```python
from build123d import *

# Parameters (mm, degrees)
F0_R     = 17.5
F0_R_2   = 15.5
F1_DEPTH = 6
F2_R     = 20
F3_DEPTH = 2
F4_SIZE  = 2.49999


# Not quite as in the source:
# - a fillet or chamfer is up to 0.001 mm smaller than in the source, because OpenCascade refuses the exact size


with BuildPart() as f1:
    # F0 (on Top) → F1 (new body)
    with BuildSketch(Plane.XY):
        Circle(F0_R)
        Circle(F0_R_2, mode=Mode.SUBTRACT)
    extrude(amount=F1_DEPTH)

    # F2 (on Top) → F3 (join)
    with BuildSketch(Plane.XY):
        Circle(F2_R)
    extrude(amount=F3_DEPTH)

    # F4 (size 2.5 in the source; OpenCascade refuses exactly that, so slightly less here)
    f4_edges = [f1.edges().sort_by_distance(p)[0] for p in [
        (-17.5, 0, 2),
    ]]
    chamfer(f4_edges, length=F4_SIZE)


solid = f1.part
```
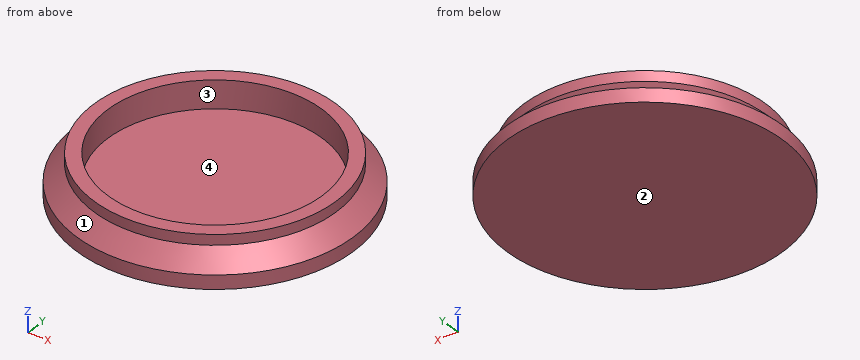
The listing builds one solid part. Answer for the finished solid, in the listing's coordinates (mm). Face numbers are marked on the shaded views. Give positions to 0.01 mm unless a question says otherwise; leave off trailing zeros. Order: outer loops, then holes, each group sorted by start corner. A loop starts at its lowest first (then second) coordinate and runs counter-clockwise, first axis right, second up. Notation, with made-up numbers: (18.25, 56.25) - (44.25, 56.25) arc R21 cw to (44.25, 69.25) - close; hole circle Ø7 at (-4, 25.25). An arc over 180 degrees is marked (long way). Answer in a Markdown table with one row per item. Add a question column.
Q1. For a pull along Y with two mould halves and no side action, classify the marked faces 1, 2, 3 and 4 as released by +Y, released by -Y, zero draft, split by the parting line, or undercut.
Q2. Find the intervals of material crossed by line 1 along Z through (x, y) = (-12, -1.5); line 2 along Y through (x, z) = (0, 3.9); line 3 along X through (y, z) = (0, 3.95), in increasing order. Write a range as [from, to].
Q3. The part is cut by section C-C (z = 3.4). Determine the outline of the cut face in (x, y), then the cut area to 3 significant figures.
Q4. Given P1, Ø6, axis at x = 11, y = -10, coming from the +Z side, flat-ended and moving along its own axis, determine where the tip first touches the part or whether it passes through.
Determined:
| question | item | result |
|---|---|---|
| 1 | face 1 | split by the parting line |
| 1 | face 2 | zero draft |
| 1 | face 3 | undercut |
| 1 | face 4 | undercut |
| 2 | line 1 | z = [0, 2] |
| 2 | line 2 | y = [-18.1, -15.5], [15.5, 18.1] |
| 2 | line 3 | x = [-18.05, -15.5], [15.5, 18.05] |
| 3 | outline | circle Ø37.2 at (0, 0); hole circle Ø31 at (0, 0) |
| 3 | area | 332 mm² |
| 4 | P1 | stops at z = 6 |
